```python
from build123d import *

# Parameters (mm, degrees)
CROQUIS1_W              = 58
CROQUIS1_H              = 12.5
CROQUIS1_R              = 1.55
SALIENTE_EXTRUIR1_DEPTH = 15
SALIENTE_EXTRUIR2_DEPTH = 15
CROQUIS2_R              = 2
CORTAR_EXTRUIR1_DEPTH   = 45.520669357
CROQUIS24_R             = 6.75
CORTAR_EXTRUIR10_DEPTH  = 5
CROQUIS25_R             = 5.25
CORTAR_EXTRUIR11_DEPTH  = 2.5
CROQUIS26_R             = 3.25
CORTAR_EXTRUIR12_DEPTH  = 7.5
TALADRO_ROSCADO_M81_D   = 6.8
CHAFL_N1_SIZE           = 4
CHAFL_N2_SIZE           = 2
CROQUIS34_R             = 5
CORTAR_EXTRUIR13_DEPTH  = 45.520669435
CHAFL_N3_SIZE           = 1
CHAFL_N3_SIZE2          = 1.732050808
CROQUIS35_R             = 7.2
CORTAR_EXTRUIR14_DEPTH  = 1


with BuildPart() as part:
    # Croquis1 → Saliente-Extruir1 (new body)
    with BuildSketch(Plane(origin=(0, 0, 0), x_dir=(1, 0, 0), z_dir=(0, 1, 0))):
        with Locations((-8, 0.25)):
            Rectangle(CROQUIS1_W, CROQUIS1_H)
        with Locations(Location((0, 0, 0), (0, 0, 270))):
            Circle(CROQUIS1_R, mode=Mode.SUBTRACT)
        with Locations(Location((-31, 0, 0), (0, 0, 270))):
            Circle(CROQUIS1_R, mode=Mode.SUBTRACT)
    extrude(amount=SALIENTE_EXTRUIR1_DEPTH)

    # Croquis5 → Saliente-Extruir2 (add)
    with BuildSketch(Plane(origin=(0, 0, 0), x_dir=(1, 0, 0), z_dir=(0, 1, 0))):
        with BuildLine():
            Line((21, 6.5), (21, 10.3))
            Line((21, 10.3), (-15.5, 10.3))
            ThreePointArc((-15.5, 10.3), (-18.473213749, 11.233854198), (-20.378524367, 13.7))
            Line((-20.378524367, 13.7), (-20.653079285, 13.7))
            ThreePointArc((-20.653079285, 13.7), (-25.099122875, 9.875702269), (-30.8, 8.5))
            Line((-30.8, 8.5), (-37, 8.5))
            Line((-37, 8.5), (-37, 6.5))
            Line((-37, 6.5), (21, 6.5))
        make_face()
    extrude(amount=SALIENTE_EXTRUIR2_DEPTH)

    # Croquis2 → Cortar-Extruir1 (cut, through all)
    with BuildSketch(Plane.XY.offset(6)):
        with Locations((-20.2, 7.5)):
            Circle(CROQUIS2_R)
    extrude(amount=-CORTAR_EXTRUIR1_DEPTH, mode=Mode.SUBTRACT)

    # Croquis24 → Cortar-Extruir10 (cut)
    with BuildSketch(Plane.XY.offset(6)):
        with Locations((-20.2, 7.5)):
            Circle(CROQUIS24_R)
    extrude(amount=-CORTAR_EXTRUIR10_DEPTH, mode=Mode.SUBTRACT)

    # Croquis25 → Cortar-Extruir11 (cut)
    with BuildSketch(Plane.XY.offset(1)):
        with Locations((-20.2, 7.5)):
            Circle(CROQUIS25_R)
    extrude(amount=-CORTAR_EXTRUIR11_DEPTH, mode=Mode.SUBTRACT)

    # Croquis26 → Cortar-Extruir12 (cut)
    with BuildSketch(Plane.XY.offset(-1.5)):
        with Locations((-20.2, 7.5)):
            Circle(CROQUIS26_R)
    extrude(amount=-CORTAR_EXTRUIR12_DEPTH, mode=Mode.SUBTRACT)

    # Taladro roscado M81 (through all)
    with Locations(Plane.XY.offset(6)):
        with Locations((6, 7.5)):
            Hole(TALADRO_ROSCADO_M81_D / 2)

    # Chaflán1
    chafl_n1_edges = [part.edges().sort_by_distance(p)[0] for p in [
        (-37, 7.5, 6),
    ]]
    chamfer(chafl_n1_edges, length=CHAFL_N1_SIZE)

    # Chaflán2
    chafl_n2_edges = [part.edges().sort_by_distance(p)[0] for p in [
        (21, 7.5, 6),
    ]]
    chamfer(chafl_n2_edges, length=CHAFL_N2_SIZE)

    # Croquis34 → Cortar-Extruir13 (cut, through all)
    with BuildSketch(Plane.XY.offset(6)):
        with Locations((-7, 7.5)):
            Circle(CROQUIS34_R)
    extrude(amount=-CORTAR_EXTRUIR13_DEPTH, mode=Mode.SUBTRACT)

    # Chaflán3
    chafl_n3_edges = [part.edges().sort_by_distance(p)[0] for p in [
        (-23.45, 7.5, -1.5),
    ]]
    chafl_n3_side = [part.faces().sort_by_distance(p)[0] for p in [
        (-25.301507576, 7.5, -1.5),
    ]]
    chamfer(chafl_n3_edges, length=CHAFL_N3_SIZE, length2=CHAFL_N3_SIZE2, reference=chafl_n3_side[0])

    # Croquis35 → Cortar-Extruir14 (cut)
    with BuildSketch(Plane.XY.offset(6)):
        with Locations((-20.2, 7.5)):
            Circle(CROQUIS35_R)
    extrude(amount=-CORTAR_EXTRUIR14_DEPTH, mode=Mode.SUBTRACT)


solid = part.part
```
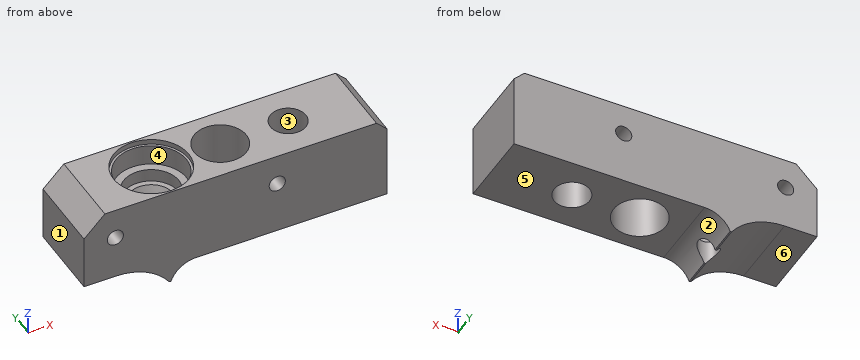
Part model, mm, in its own coordinate system. Face numbers are marked on the shaded views. A direction names the side the tool comes from. Round coordinates to 2 decimals unless told otherwise and drop trailing zeros. Order: outer loops, then holes, each group sorted by start corner. A loop starts at its lowest first (then second) coordinate and runs counter-clockwise, first axis right, second up. Notation, with made-up numbers: M 33,21 L 75,21 A33 ccw 75,51 Z; hole C 86,64 d4. An arc over 180 degrees is marked long. Put each result on its own line as item: value. Start each with the question number.
1. Two-plate mould, pull along X, no slides. Class the marked faces 1, 2 and 3: +X half, -X half, draft (parallel to the pull), parting line (faces both ways), or undercut.
2. Tool access for the marked faces 4, 5 and 6: list every direction of +Z, -Z, +X, -X, +Y, -Y with a clear straight run to the whole face (end or side of a thin tool).
3. Slice it at B-B on x = 6. List the corners of the cut face in (y, z), then the cut area to 3 significant figures.
4. Slice it at A-A on z = 0. List the corners of the cut face in (x, y).
5. Slice it at C-C on y = 8.5. State how many separate pieces and enclosed holes the cut face has, then the cut area to 3 significant figures.
6. Drop flat-ended pins along their axis: pin 1 (2 mm diameter, centred on x = 10, z = -11, fed in from -Y); pin 2 (1 mm diameter, centred on x = -24.5, y = 6.5, fed in from -Z); pin 3 (3 mm diameter, centred on x = -20.5, y = 7, fed in from +Z); pin 4 (3 mm diameter, centred on x = -33, y = 5.5, fed in from -Z). Give the stop position or say it passes through.
7. Slice it at D-D on x = 0. List the corners of the cut face in (y, z), then the cut area to 3 significant figures.
8. Drill centre lines: probe 1 along Y at (x, z) = (-20.2, 5.5); probe 2 along Y at (x, z) = (-7, -1.25); probe 3 along X at (y, z) = (4, 0). Where is each one in solid material? Low to high. Write a range as [from, to].
Findings:
1. face 1: -X half
1. face 2: +X half
1. face 3: undercut
2. face 4: +Z
2. face 5: -Z, +X, +Y, -Y
2. face 6: -Z, -X, +Y, -Y
3. outline: M 0,-10.3 L 4.1,-10.3 L 4.1,6 L 0,6 Z; M 10.9,-10.3 L 15,-10.3 L 15,6 L 10.9,6 Z
3. area: 134 mm2
4. outline: M -37,0 L -32.55,0 L -32.55,15 L -37,15 Z; M -29.45,0 L -1.55,0 L -1.55,15 L -29.45,15 Z; M 1.55,0 L 21,0 L 21,15 L 1.55,15 Z; hole C -20.2,7.5 d10.5; hole C -7,7.5 d10; hole C 6,7.5 d6.8
5. separate pieces: 4
5. enclosed holes: 2
5. area: 492 mm2
6. pin 1: y = 0
6. pin 2: z = -10.51
6. pin 3: z = -9
6. pin 4: z = -8.5
7. outline: M 0,-10.3 L 15,-10.3 L 15,-1.55 L 0,-1.55 Z; M 0,1.55 L 15,1.55 L 15,6 L 0,6 Z
7. area: 198 mm2
8. probe 1: [0, 0.3], [14.7, 15]
8. probe 2: [0, 2.5], [12.5, 15]
8. probe 3: [-37, -32.55], [-29.45, -24.11], [-16.29, -10.57], [-3.43, -1.55], [1.55, 21]
